Build history of the part. All positions in model axes, mm. Face numbers are marked on the shaded views. A direction names the side the tool comes from. Round coordinates to 2 decimals unless told otherwise and drop trailing zeros. Loops run counter-clockwise (first coordinate to the right, second up) from the corner with the lowest first, then second, coordinate; pieces in that order, holes last. Notation, with made-up numbers: M 17.25,42 L 53.25,42 A25 ccw 53.25,63 Z; hole C 80,-29 d11. An arc over 180 degrees is marked long. Write each question's results on one line, items separated by ' | '. Start each with the question number.
```python
from build123d import *

# Parameters (mm, degrees)
BOSS_EXTRUDE1_DEPTH = 10
SKETCH2_R           = 2.5
CUT_EXTRUDE1_DEPTH  = 36.832945734
FILLET1_R           = 3
SKETCH3_R           = 2
CUT_EXTRUDE2_DEPTH  = 26.475478406


with BuildPart() as part:
    # Sketch1 → Boss-Extrude1 (new body)
    with BuildSketch(Plane(origin=(0, 0, 0), x_dir=(1, 0, 0), z_dir=(0, 1, 0))):
        Polygon((-18, 0), (18, 0), (18, 5), (10, 5), (10, 20), (5, 20), (5, 5), (-5, 5), (-5, 20), (-10, 20), (-10, 5), (-18, 5), align=None)
    extrude(amount=BOSS_EXTRUDE1_DEPTH)

    # Sketch2 → Cut-Extrude1 (cut, through all)
    with BuildSketch(Plane(origin=(10, 0, 0), x_dir=(0, 0, -1), z_dir=(1, 0, 0))):
        with Locations((15, 5)):
            Circle(SKETCH2_R)
    extrude(amount=-CUT_EXTRUDE1_DEPTH, mode=Mode.SUBTRACT)

    # Fillet1
    fillet1_edges = [part.edges().sort_by_distance(p)[0] for p in [
        (18, 0, -2.5),
        (7.5, 10, -20),
        (-18, 0, -2.5),
        (-7.5, 0, -20),
        (7.5, 0, -20),
        (-7.5, 10, -20),
        (-18, 10, -2.5),
        (18, 10, -2.5),
    ]]
    fillet(fillet1_edges, radius=FILLET1_R)

    # Sketch3 → Cut-Extrude2 (cut, through all)
    with BuildSketch(Plane(origin=(0, 0, -5), x_dir=(-1, 0, 0), z_dir=(0, 0, -1))):
        with Locations((14, 5)):
            Circle(SKETCH3_R)
        with Locations((-14, 5)):
            Circle(SKETCH3_R)
    extrude(amount=-CUT_EXTRUDE2_DEPTH, mode=Mode.SUBTRACT)


solid = part.part
```
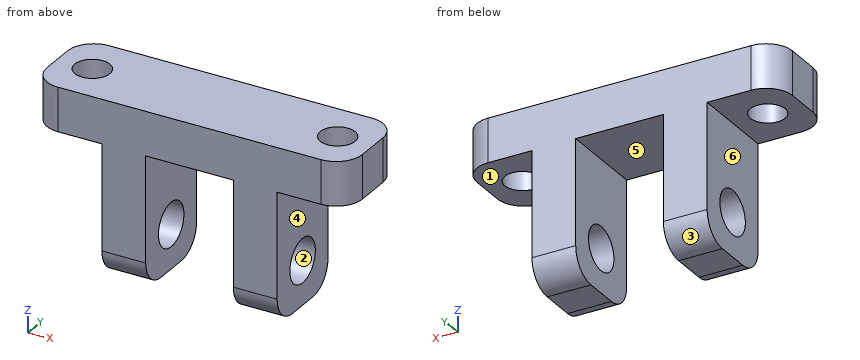
Item 1: Drop flat-ended pins along their axis: pin 1 (3 mm diameter, centred on x = 1.5, y = 3.5, fed in from -Z); pin 2 (3 mm diameter, centred on y = 4.5, z = -9, fed in from +X). Give the stop position or say it passes through.
Item 2: Mould opens along Y. For the marked faces 1, 2 and 3 say: released by +Y, released by -Y, zero draft, split by the parting line, or undercut.
Item 3: Saw through at C-C, the plane y = 5. Give the cut face in (x, z).
Item 4: Saw through at A-A, the plane z = -9.25. Give the cut face in (x, y).
Item 5: Saw through at D-D, the plane x = -7. Give the cut face in (y, z).
Item 6: Tool access for the marked faces 4, 5 and 6: list every direction of +Z, -Z, +X, -X, +Y, -Y with a clear straight run to the whole face (end or side of a thin tool).
Item 7: Drill centre lines: line 1 along X through (y, z) = (3, -11.75); line 2 along Y through (x, z) = (-14, -2); line 3 along X through (y, z) = (6.5, -4). Where is each one in solid material? Low to high. Write a range as [from, to].
Item 8: Saw through at B-B, the plane x = -14. Give the cut face in (y, z), then the cut area to 3 significant figures.
Working result:
1) pin 1: stops at z = -5 | pin 2: stops at x = 10
2) face 1: zero draft | face 2: undercut | face 3: released by +Y
3) outline: M -18,-5 L -16,-5 L -16,0 L -18,0 Z; M -12,-5 L -10,-5 L -10,-12.5 L -5,-12.5 L -5,-5 L 5,-5 L 5,-12.5 L 10,-12.5 L 10,-5 L 12,-5 L 12,0 L -12,0 Z; M -10,-20 L -5,-20 L -5,-17.5 L -10,-17.5 Z; M 5,-20 L 10,-20 L 10,-17.5 L 5,-17.5 Z; M 16,-5 L 18,-5 L 18,0 L 16,0 Z
4) outline: M -10,0 L -5,0 L -5,10 L -10,10 Z; M 5,0 L 10,0 L 10,10 L 5,10 Z
5) outline: M 0,-17 A3 ccw 3,-20 L 7,-20 A3 ccw 10,-17 L 10,0 L 0,0 Z; hole C 5,-15 d5
6) face 4: -Z, +X, +Y, -Y | face 5: -Z, +Y, -Y | face 6: -Z, -X, +Y, -Y
7) line 1: x = [-10, -5], [5, 10] | line 2: y = [0, 3], [7, 10] | line 3: x = [-18, -15.32], [-12.68, 12.68], [15.32, 18]
8) outline: M 0,-5 L 3,-5 L 3,0 L 0,0 Z; M 7,-5 L 10,-5 L 10,0 L 7,0 Z | area: 30.0 mm²
